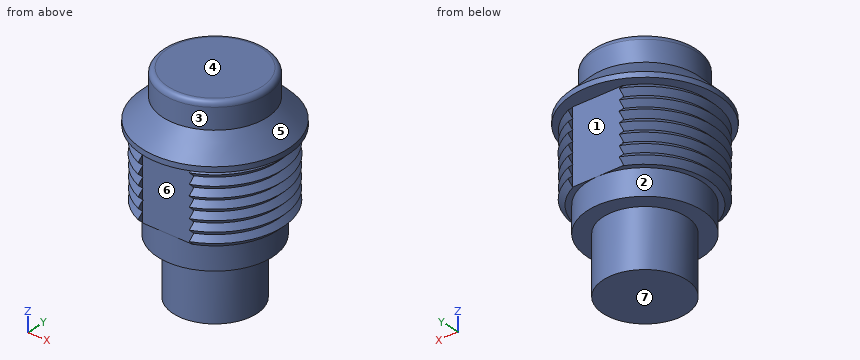
```python
from build123d import *

# Parameters (mm, degrees)
F2_W      = 6
F2_H      = 7
F10_SIZE2 = 1.99999
F10_SIZE  = 1.99999
F11_R     = 0.5
F12_W     = 5
F12_H     = 3.4022161548
F12_H_2   = 4.2761773802
F13_DEPTH = 15


# Not quite as in the source:
# - a fillet or chamfer is up to 0.001 mm smaller than in the source, because OpenCascade refuses the exact size


with BuildPart() as f1:
    # F0 (on Front) → F1 (revolve)
    with BuildSketch(Plane.XZ):
        Polygon((0, 8), (0, 0), (4, 0), (4, 5.5), (5.5, 5.5), (5.5, 8), align=None)
    revolve(axis=Axis((0, 0, 8.8947357469), (0, 0, 1)))

    # F2 (on Front) → F3 (revolve)
    with BuildSketch(Plane.XZ):
        with Locations((3, 11.5)):
            Rectangle(F2_W, F2_H)
    revolve(axis=Axis((0, 0, 12.8918935508), (0, 0, 1)))

    # F6 (on Front) → F7 (revolve)
    with BuildSketch(Plane.XZ):
        Polygon((-6.5108180568, 8.5108180568), (-6, 8), (0, 8), (0, 15), (-5.9985076077, 15), (-6.5, 14.5), (-6, 14), (-6.5, 13.5), (-6, 13), (-6.532786414, 12.5), (-6, 12), (-6.5, 11.5), (-6, 11), (-6.5, 10.5), (-6, 10), (-6.5, 9.5), (-6.0216361135, 9), align=None)
    revolve(axis=Axis((0, 0, 9.6160949171), (0, 0, 1)))

    # F8 (on Front) → F9 (revolve)
    with BuildSketch(Plane.XZ):
        Polygon((-7, 15), (0, 15), (0, 20), (-5, 20), (-5, 17.5), (-7, 17.5), align=None)
    revolve(axis=Axis((0, 0, 18.9704594016), (0, 0, 1)))

    # F10 (size 2 and 2 in the source; OpenCascade refuses exactly that, so slightly less here)
    f10_edges = [f1.edges().sort_by_distance(p)[0] for p in [
        (7, 0, 17.5),
    ]]
    chamfer(f10_edges, length=F10_SIZE, length2=F10_SIZE2)

    # F11
    f11_edges = [f1.edges().sort_by_distance(p)[0] for p in [
        (5, 0, 20),
    ]]
    fillet(f11_edges, radius=F11_R)

    # F12 (on Top) → F13 (cut, through all)
    with BuildSketch(Plane.XY):
        with Locations((0, 7.2011080774)):
            Rectangle(F12_W, F12_H)
        with Locations((0, -7.6380886901)):
            Rectangle(F12_W, F12_H_2)
    extrude(amount=F13_DEPTH, mode=Mode.SUBTRACT)


solid = f1.part
```
Part model, mm, in its own coordinate system. Face numbers are marked on the shaded views. A direction names the side the tool comes from. Round coordinates to 2 decimals unless told otherwise and drop trailing zeros. Loops run counter-clockwise (first coordinate to the right, second up) from the corner with the lowest first, then second, coordinate; pieces in that order, holes last.
1. Slice it at A-A (z = 7.75). Give the cut face in (x, y).
Solutions:
outline: circle Ø11 at (0, 0)
2. Flat gauge pins, fed straight in: pin 1 (4 mm diameter, centred on y = 0, z = 16, fed in from +X); pin 2 (0.6 mm diameter, centred on y = 6, z = 14.5, fed in from +X); pin 3 (4 mm diameter, centred on x = 3.5, z = 14, fed in from +Y); pin 4 (4 mm diameter, centred on x = -1, z = 3, fed in from +Y). Where does each tip first touch, or does it go through?
Solutions:
pin 1: stops at x = 7
pin 2: stops at x = 3.12
pin 3: stops at y = 6.77
pin 4: stops at y = 4
3. Two-plate mould, pull along X, no slides. Class the marked faces 5, 6 and 7: pulls with the +X half, pulls with the -X half, needs draft (parallel to the pull), parting line crosses it, or undercut.
Solutions:
face 5: parting line crosses it
face 6: undercut
face 7: needs draft
4. Drill centre lines: line 1 along Z through (x, y) = (-2.5, 3.75); line 2 along Y through (x, z) = (0.25, 11.75); line 3 along X through (y, z) = (-3, 17). Where is each one in solid material? Low to high.
Solutions:
line 1: z = 5.5 to 20
line 2: y = -5.5 to 5.5
line 3: x = -4.61 to 4.61
5. 3-axis set-ups, long thin cutter, end or side, ignore diameter. For the marked faces 1, 2, 3 and 4: which of +Z, -Z, +X, -X, +Y, -Y reach the whole face in a straight line?
Solutions:
face 1: -Z, +Y
face 2: -Z
face 3: +Z
face 4: +Z, +X, -X, +Y, -Y
